```python
from build123d import *

# Parameters (mm, degrees)
SKETCH1_W           = 60
SKETCH1_H           = 30
BOSS_EXTRUDE1_DEPTH = 4
SHELL1_T            = -2
SKETCH2_R           = 2
BOSS_EXTRUDE2_DEPTH = 10
FILLET1_R           = 1
CHAMFER1_SIZE       = 1


with BuildPart() as part:
    # Sketch1 → Boss-Extrude1 (new body)
    with BuildSketch(Plane(origin=(0, 0, 0), x_dir=(1, 0, 0), z_dir=(0, 1, 0))):
        Rectangle(SKETCH1_W, SKETCH1_H)
    extrude(amount=BOSS_EXTRUDE1_DEPTH)

    # Shell1
    shell1_openings = [part.faces().sort_by_distance(p)[0] for p in [
        (0, 0, 0),
    ]]
    offset(amount=SHELL1_T, openings=shell1_openings, kind=Kind.INTERSECTION)

    # Sketch2 → Boss-Extrude2 (add)
    with BuildSketch(Plane.XZ.offset(-2)):
        with Locations((-15, 0)):
            Circle(SKETCH2_R)
        with Locations((15, 0)):
            Circle(SKETCH2_R)
    extrude(amount=BOSS_EXTRUDE2_DEPTH)

    # Fillet1
    fillet1_edges = [part.edges().sort_by_distance(p)[0] for p in [
        (-17, -8, 0),
        (13, -8, 0),
    ]]
    fillet(fillet1_edges, radius=FILLET1_R)

    # Chamfer1
    chamfer1_edges = [part.edges().sort_by_distance(p)[0] for p in [
        (-30, 4, 0),
        (0, 4, 15),
        (30, 4, 0),
        (0, 4, -15),
    ]]
    chamfer(chamfer1_edges, length=CHAMFER1_SIZE)


solid = part.part
```
Check sheet for the modelled part. Datum: model origin and axes. Units: mm. A direction names the side the tool comes from. Coordinates: 2 decimals unless noted, no trailing zeros. Order: outer loops, then holes, each group sorted by start corner. A loop starts at its lowest first (then second) coordinate and runs counter-clockwise, first axis right, second up. Notation, with made-up numbers: (5, 60.25) -> (37, 60.25) arc R33 cw to (37, 98.25) -> close; hole circle Ø7 at (18.5, 56.5). An arc over 180 degrees is marked (long way). Write item = value, one per line. Start each with the question number.
1) Cross-section at B-B (x = -11.5). Enter the section's corners in (y, z), then the cut area to 3 significant figures.
2) Cross-section at C-C (y = -2.75). Enter the section's corners in (x, z).
3) Material ranges on L1, parallel to X at y = 0.5, z = -7.5; L2, parallel to Z at x = -24, y = 1; L3, parallel to Y at x = 24.5, z = -1.5, recorded low to high.
4) Cross-section at A-A (z = 6.5). Enter the section's corners in (x, y).
5) Mould release check, pull along Z, two halves, no side actions. Record for faces 1 (the flat face through (0, 1, -13)), 2 (the flat face through (0, 1, -15)), 3 (the flat face through (-28, 1, 0)), 4 (the flat face through (-2.4, 0, 13.3)): +Z half, -Z half, draft (parallel to the pull), parting line (faces both ways), or undercut.
6) Go/stop test with flat-tipped pins: P1, Ø15, axis at x = 6, z = 2, coming from the -Y side; P2, Ø5, axis at x = 1.5, z = 3.5, coming from the -Y side; P3, Ø1, axis at x = 15, y = -1, coming from the +Z side. Record where each tip stops, or that it passes through.
7) Access from +Z, -Z, +X, -X, +Y, -Y to the whole of each face (thin tool, end or side, straight path). Record for faces 5 (the flat face through (0, 2, 0)), 6 (the flat face through (0, 1, 15)).
Ans:
q1.outline = (0, -15) -> (3, -15) -> (4, -14) -> (4, 14) -> (3, 15) -> (0, 15) -> (0, 13) -> (2, 13) -> (2, -13) -> (0, -13) -> close
q1.area = 67.0 mm²
q2.outline = circle Ø4 at (-15, 0); circle Ø4 at (15, 0)
q3.L1 = -30 to -28, 28 to 30
q3.L2 = -15 to -13, 13 to 15
q3.L3 = 2 to 4
q4.outline = (-30, 0) -> (-28, 0) -> (-28, 2) -> (28, 2) -> (28, 0) -> (30, 0) -> (30, 3) -> (29, 4) -> (-29, 4) -> (-30, 3) -> close
q5.face_1 = undercut
q5.face_2 = -Z half
q5.face_3 = undercut
q5.face_4 = draft
q6.P1 = -7.69
q6.P2 = 2
q6.P3 = 2
q7.face_5 = -Y
q7.face_6 = +Z, +X, -X, +Y, -Y
